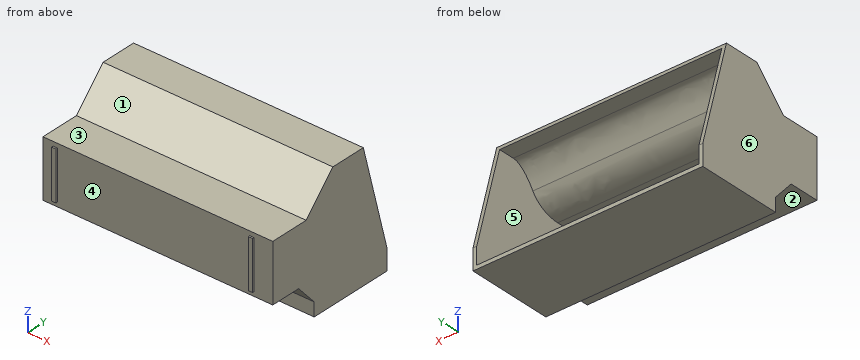
from build123d import *

# Parameters (mm, degrees)
SKIZZE1_W                       = 800
SKIZZE1_H                       = 200
AUFSATZ_LINEAR_AUSTRAGEN1_DEPTH = 274
SKIZZE2_W                       = 15
SKIZZE2_H                       = 170
AUFSATZ_LINEAR_AUSTRAGEN2_DEPTH = 6
AUFSATZ_LINEAR_AUSTRAGEN4_DEPTH = 800
SKIZZE8_W                       = 774
SKIZZE8_H                       = 408.84
SCHNITT_LINEAR_AUSTRAGEN3_DEPTH = 217
SKIZZE9_W                       = 774
SKIZZE9_H                       = 294
SCHNITT_LINEAR_AUSTRAGEN4_DEPTH = 71
SKIZZE10_W                      = 774
SKIZZE10_H                      = 174
SCHNITT_LINEAR_AUSTRAGEN5_DEPTH = 170
VERRUNDUNG1_SIZE                = 115
VERRUNDUNG1_SIZE_2              = 95
VERRUNDUNG2_SIZE                = 95
VERRUNDUNG2_SIZE_2              = 115
VERRUNDUNG3_START               = -371
VERRUNDUNG3_DEPTH               = 776


with BuildPart() as part:
    # Skizze1 → Aufsatz-Linear austragen1 (new body)
    with BuildSketch(Plane(origin=(0, 0, 0), x_dir=(1, 0, 0), z_dir=(0, 1, 0))):
        with Locations((17.371106882, 37.147335423)):
            Rectangle(SKIZZE1_W, SKIZZE1_H)
    extrude(amount=AUFSATZ_LINEAR_AUSTRAGEN1_DEPTH)

    # Skizze2 → Aufsatz-Linear austragen2 (add)
    with BuildSketch(Plane(origin=(0, 0, 0), x_dir=(-1, 0, 0), z_dir=(0, -1, 0))):
        with Locations((340.128893118, 37.147335423)):
            Rectangle(SKIZZE2_W, SKIZZE2_H)
        with Locations((-344.871106882, 37.147335423)):
            Rectangle(SKIZZE2_W, SKIZZE2_H)
    extrude(amount=AUFSATZ_LINEAR_AUSTRAGEN2_DEPTH)

    # Skizze7 → Aufsatz-Linear austragen4 (add)
    with BuildSketch(Plane.ZY.offset(382.628893118)):
        Polygon((-137.147335423, 106.095397632), (-209.709609496, 169.941826261), (-257.147335423, 169.941826261), (-257.147335423, 468.401582256), (-184.807335423, 468.401582256), (177.692664577, 371.27), (177.692664577, 246.474221491), (62.852664577, 137), align=None)
    extrude(amount=-AUFSATZ_LINEAR_AUSTRAGEN4_DEPTH)

    # Skizze8 → Schnitt-Linear austragen3 (cut)
    with BuildSketch(Plane(origin=(0, 468.401582256, 0), x_dir=(1, 0, 0), z_dir=(0, 1, 0))):
        with Locations((17.371106882, 39.727335423)):
            Rectangle(SKIZZE8_W, SKIZZE8_H)
    extrude(amount=-SCHNITT_LINEAR_AUSTRAGEN3_DEPTH, mode=Mode.SUBTRACT)

    # Skizze9 → Schnitt-Linear austragen4 (cut)
    with BuildSketch(Plane(origin=(0, 251.401582256, 0), x_dir=(1, 0, 0), z_dir=(0, 1, 0))):
        with Locations((17.371106882, 97.147335423)):
            Rectangle(SKIZZE9_W, SKIZZE9_H)
    extrude(amount=-SCHNITT_LINEAR_AUSTRAGEN4_DEPTH, mode=Mode.SUBTRACT)

    # Skizze10 → Schnitt-Linear austragen5 (cut)
    with BuildSketch(Plane(origin=(0, 180.401582256, 0), x_dir=(1, 0, 0), z_dir=(0, 1, 0))):
        with Locations((17.371106882, 37.147335423)):
            Rectangle(SKIZZE10_W, SKIZZE10_H)
    extrude(amount=-SCHNITT_LINEAR_AUSTRAGEN5_DEPTH, mode=Mode.SUBTRACT)

    # Verrundung1
    # a fillet whose section is not a circle: 115, 95 mm, written as the material it takes off along each edge
    with BuildSketch(Plane(origin=(-369.628893118, 180.401582256, -124.147335423), x_dir=(0, -1, 0), z_dir=(1, 0, 0))) as verrundung1_piece_1:
        with BuildLine():
            Bezier((VERRUNDUNG1_SIZE, 0), (0, 0), (0, VERRUNDUNG1_SIZE_2), weights=[1, 0.707106781, 1])
            Line((0, VERRUNDUNG1_SIZE_2), (0, 0))
            Line((0, 0), (VERRUNDUNG1_SIZE, 0))
        make_face()
    extrude(amount=774, mode=Mode.SUBTRACT)

    # Verrundung2
    # a fillet whose section is not a circle: 115, 95 mm, written as the material it takes off along each edge
    with BuildSketch(Plane(origin=(-369.628893118, 251.401582256, 49.852664577), x_dir=(0, 0, 1), z_dir=(1, 0, 0))) as verrundung2_piece_1:
        with BuildLine():
            Bezier((VERRUNDUNG2_SIZE, 0), (0, 0), (0, VERRUNDUNG2_SIZE_2), weights=[1, 0.707106781, 1])
            Line((0, VERRUNDUNG2_SIZE_2), (0, 0))
            Line((0, 0), (VERRUNDUNG2_SIZE, 0))
        make_face()
    extrude(amount=774, mode=Mode.SUBTRACT)

    # Verrundung3: read off the stored shape, not the designer's step
    # Verrundung3 outline → Verrundung3 (add)
    with BuildSketch(Plane.YZ.offset(VERRUNDUNG3_START)):
        with BuildLine():
            add(Edge.make_bspline(
                [(251.401582257, 144.852664577), (251.401582257, 121.417687853), (238.208250652, 100.671279991)],
                knots=[0, 0, 0, 0.316521674, 0.316521674, 0.316521674], degree=2, weights=[1, 0.907292948, 0.873273479]))
            add(Edge.make_bspline(
                [(238.208250652, 100.671279991), (278.921580984, 164.69266458), (318.371713455, 164.692664577)],
                knots=[0, 0, 0, 1, 1, 1], degree=2, weights=[1, 0.876532088, 1]))
            Line((318.371713455, 164.692664577), (251.401582251, 164.692664573))
            Line((251.401582251, 164.692664573), (251.401582257, 144.852664577))
        make_face()
        with BuildLine():
            Line((180.401582251, -244.147335419), (250.535882306, -244.147335423))
            add(Edge.make_bspline(
                [(250.535882306, -244.147335423), (208.142607951, -244.147335414), (168.747010016, -177.475177999)],
                knots=[0, 0, 0, 1, 1, 1], degree=2, weights=[1, 0.868537314, 1]))
            add(Edge.make_bspline(
                [(168.747010016, -177.475177999), (180.401582257, -197.199094267), (180.401582257, -219.147335423)],
                knots=[0.70180493, 0.70180493, 0.70180493, 1, 1, 1], degree=2, weights=[0.877409678, 0.912660686, 1]))
            Line((180.401582257, -219.147335423), (180.401582251, -244.147335419))
        make_face()
    extrude(amount=VERRUNDUNG3_DEPTH)


solid = part.part
Source: CAD feature listing. Evaluate the final solid. Frame: model axes, mm. Face numbers are marked on the shaded views. A direction names the side the tool comes from. Give positions to 0.01 mm unless a question says otherwise; leave off trailing zeros. Write each loop counter-clockwise with the first axis right and the second up, starting at its lowest first coordinate (ties: lowest second). Pieces come first, ordered by that corner, then holes. Notation, with made-up numbers: M -26.75,-26.75 L -22.75,-26.75 A30 ccw -22.75,2.25 Z; hole C 42,22.25 d6. An arc over 180 degrees is marked long. Return JSON: item names as keys, results as strings. Group by question number.
1) Cut plane A-A, the plane z = -38.5. Output: boundary loops of the cut face in (x, y), plus the area to 3 significant figures.
2) Pull-direction query (X, two-part tool) for the marked faces 3, 4, 5 and 6; classes: pulls with the +X half, pulls with the -X half, needs draft (parallel to the pull), parting line crosses it, or undercut.
3) Set-up query: the marked faces 1 and 2. Return all of +Z, -Z, +X, -X, +Y, -Y with unobstructed straight access to the full face (end or side cutting, diameter ignored); none if empty.
4) Material intervals for line 1 along X through (y, z) = (175.5, 37); line 2 along Z through (x, y) = (-147, 359); line 3 along Y through (x, z) = (-170, 21), sorted ascending. Write a range as [from, to].
5) Cut plane B-B, the plane y = 395.5. Output: boundary loops of the cut face in (x, z).
6) Pin query (flat end, axial travel): P1, Ø10, axis at x = 217.5, z = -148.5, coming from the +Y side; P2, Ø6.5, axis at y = -2, z = -22.5, coming from the +X side; P3, Ø6, axis at x = -19, y = 97, coming from the +Z side; P4, Ø3, axis at x = 346.5, y = -2, coming from the +Z side. Return the tip coordinate at first contact, or that it passes through.
Recorded:
{
 "1": {"outline": "M -382.63,0 L -347.63,0 L -347.63,-6 L -332.63,-6 L -332.63,0 L 337.37,0 L 337.37,-6 L 352.37,-6 L 352.37,0 L 417.37,0 L 417.37,429.2 L 404.37,429.2 L 404.37,10.4 L -369.63,10.4 L -369.63,429.2 L -382.63,429.2 Z", "area": "19,400 mm²"},
 "2": {"face 3": "needs draft", "face 4": "undercut", "face 5": "undercut", "face 6": "pulls with the -X half"},
 "3": {"face 1": "+Z, +X, -X, -Y", "face 2": "-Z, +X, -X, -Y"},
 "4": {"line 1": "x = [-382.63, -369.63], [404.37, 417.37]", "line 2": "z = [-257.15, -244.15], [164.69, 177.69]", "line 3": "y = [0, 10.4]"},
 "5": {"outline": "M -382.63,-257.15 L 417.37,-257.15 L 417.37,87.27 L 404.37,87.27 L 404.37,-244.15 L -369.63,-244.15 L -369.63,87.27 L -382.63,87.27 Z"},
 "6": {"P1": "stops at y = 148.53", "P2": "stops at x = 417.37", "P3": "stops at z = 62.85", "P4": "stops at z = 47.85"}
}
